```python
from build123d import *

# Parameters (mm, degrees)
SKETCH1_W           = 10
SKETCH1_H           = 5
BOSS_EXTRUDE1_DEPTH = 10
CUT_EXTRUDE1_REACH  = 14.247
SKETCH2_R           = 3
SKETCH3_W           = 20
SKETCH3_H           = 5
SKETCH3_R           = 1.6
BOSS_EXTRUDE2_DEPTH = 2
FILLET1_R           = 5


with BuildPart() as part:
    # Sketch1 → Boss-Extrude1 (new body)
    with BuildSketch(Plane(origin=(0, 0, 0), x_dir=(1, 0, 0), z_dir=(0, 1, 0))):
        Rectangle(SKETCH1_W, SKETCH1_H)
    extrude(amount=-BOSS_EXTRUDE1_DEPTH)

    # Sketch2 → Cut-Extrude1 (cut, up to next)
    with BuildSketch(Plane(origin=(0, 0, -2.5), x_dir=(-1, 0, 0), z_dir=(0, 0, -1)), mode=Mode.PRIVATE) as cut_extrude1_sk1:
        with Locations((0, -5.5)):
            Circle(SKETCH2_R)
    cut_extrude1_tool1 = extrude(cut_extrude1_sk1.sketch, amount=-CUT_EXTRUDE1_REACH, mode=Mode.PRIVATE) & part.part
    add(cut_extrude1_tool1.solids().sort_by_distance((0, -5.5, -2.5))[0], mode=Mode.SUBTRACT)

    # Sketch3 → Boss-Extrude2 (add)
    with BuildSketch(Plane(origin=(0, 0, 0), x_dir=(1, 0, 0), z_dir=(0, 1, 0))):
        Rectangle(SKETCH3_W, SKETCH3_H)
        with Locations(Location((-7.5, 0, 0), (0, 0, 270))):
            Circle(SKETCH3_R, mode=Mode.SUBTRACT)
        with Locations(Location((7.5, 0, 0), (0, 0, 270))):
            Circle(SKETCH3_R, mode=Mode.SUBTRACT)
    extrude(amount=-BOSS_EXTRUDE2_DEPTH)

    # Fillet1
    fillet1_edges = [part.edges().sort_by_distance(p)[0] for p in [
        (-5, -10, 0),
        (5, -10, 0),
    ]]
    fillet(fillet1_edges, radius=FILLET1_R - 0.0001)  # a hair under: the kernel refuses the full size


solid = part.part
```
Geometry: final body of the model. Coordinates: model frame, mm. A direction names the side the tool comes from. Coordinates: 2 decimals unless noted, no trailing zeros. Order: outer loops, then holes, each group sorted by start corner. A loop starts at its lowest first (then second) coordinate and runs counter-clockwise, first axis right, second up. Notation, with made-up numbers: M 37,-7.5 L 86,-7.5 A19 cw 86,25.5 Z; hole C 18.5,-32.75 d6. An arc over 180 degrees is marked long. Answer as CSV lines item,"result".
Q1. Section C-C on y = -5.5. Return the cut outline in (x, z).
Answers:
outline,"M -4.97,-2.5 L -3,-2.5 L -3,2.5 L -4.97,2.5 Z; M 3,-2.5 L 4.97,-2.5 L 4.97,2.5 L 3,2.5 Z"
Q2. Section A-A on z = 0. Count the separate pieces of the cut face and the enclosed holes in it, and give its area (3 significant figures).
Answers:
separate pieces,"3"
enclosed holes,"1"
area,"68.2 mm^2"
Q3. Draft query along X for faces 4 (the flat face through (5, -3, 0)), 5 (the cylindrical face through (5.94, -0.99, -0.35)), 6 (the cylindrical face through (-4, -8, 0)), 7 (the cylindrical face through (-9.06, -0.99, -0.35)). Return one class per face: pulls with the +X half, pulls with the -X half, needs draft (parallel to the pull), parting line crosses it, or undercut.
Answers:
face 4,"pulls with the +X half"
face 5,"undercut"
face 6,"pulls with the -X half"
face 7,"undercut"
Q4. Section B-B on x = -7.5. Return the cut outline in (y, z).
Answers:
outline,"M -2,-2.5 L 0,-2.5 L 0,-1.6 L -2,-1.6 Z; M -2,1.6 L 0,1.6 L 0,2.5 L -2,2.5 Z"
Q5. First-contact query: P1, Ø0.9, axis at y = -3.5, z = -1, coming from the +X side; P2, Ø2, axis at x = -1.5, z = 1, coming from the -Y side; P3, Ø5, axis at x = 0, y = -5.5, coming from the +Z side; P4, Ø3, axis at y = -7.5, z = 0, coming from the +X side. Flat tips, straight axial feed; report the tip coordinate or a pass-through.
Answers:
P1,"stops at x = 5"
P2,"stops at y = -9.97"
P3,"passes through"
P4,"stops at x = 4.9"
Q6. Set-up query: faces 1 (the flat face through (-5, -3, 0)), 2 (the flat face through (-10, -1, 0)), 3 (the flat face through (6, -2, -1)). Return all of +Z, -Z, +X, -X, +Y, -Y with unobstructed straight access to the full face (end or side cutting, diameter ignored); none if empty.
Answers:
face 1,"+Z, -Z, -X, -Y"
face 2,"+Z, -Z, -X, +Y, -Y"
face 3,"+Z, -Z, +X, -Y"
Q7. Line query: probe 1 along X at (y, z) = (-1.55, 0); probe 2 along X at (y, z) = (-0.25, 0.7); probe 3 along Y at (x, z) = (-7.5, 1.9). Output: solid intervals per line, ascending. Write a range as [from, to].
Answers:
probe 1,"x = [-10, -9.1], [-5.9, 5.9], [9.1, 10]"
probe 2,"x = [-10, -8.94], [-6.06, 6.06], [8.94, 10]"
probe 3,"y = [-2, 0]"
